Geometry check sheet. Reference: the model listing, model coordinates, mm. Give positions to 0.01 mm unless a question says otherwise; leave off trailing zeros. Loops run counter-clockwise (first coordinate to the right, second up) from the corner with the lowest first, then second, coordinate; pieces in that order, holes last. Notation, with made-up numbers: (81, 36) - (86, 36) arc R29 ccw to (86, 62) - close; hole circle Ø2 at (89, 58). An arc over 180 degrees is marked (long way). Use a Markdown table: item, result. Add a question column.
1. Cross-section at B-B on y = 2.55. Enter the section's corners in (x, z).
2. Draft check along Y on faces 1 (the flat face through (11.999, 1, 12)), 2 (the cylindrical face through (6.7, 8.06, 12.32)). Enter one of: pulls with the +Y half, pulls with the -Y half, needs draft (parallel to the pull), parting line crosses it, or undercut.
3. Cross-section at A-A on x = 2.25. Enter the section's corners in (y, z), and give its area (3 significant figures).
4. Depth check by flat-ended pin: P1, Ø12, axis at x = 2.5, y = 9, coming from the -Z side; P2, Ø0.9, axis at x = 4.75, y = 5.05, coming from the -Z side. Enter the tip coordinate at first touch or a pass-through.
5. Cross-section at C-C on z = 14.5. Count the separate pieces of the cut face and the enclosed holes in it, and give its area (3 significant figures).
from build123d import *

# Parameters (mm, degrees)
F0_W     = 22
F0_H     = 22
F0_R     = 0.75
F1_DEPTH = 25


with BuildPart() as f1:
    # F0 (on Top) → F1 (new body)
    with BuildSketch(Plane.XY):
        with Locations((0.99929, 1.25)):
            Rectangle(F0_W, F0_H)
        with Locations((-5.25, -4.95)):
            Circle(F0_R, mode=Mode.SUBTRACT)
        with Locations((-2.75, -4.95)):
            Circle(F0_R, mode=Mode.SUBTRACT)
        with Locations((-0.25, -4.95)):
            Circle(F0_R, mode=Mode.SUBTRACT)
        with Locations((-5.25, -2.45)):
            Circle(F0_R, mode=Mode.SUBTRACT)
        with Locations((-5.25, 0.05)):
            Circle(F0_R, mode=Mode.SUBTRACT)
        with Locations((-2.75, -2.45)):
            Circle(F0_R, mode=Mode.SUBTRACT)
        with Locations((-0.25, -2.45)):
            Circle(F0_R, mode=Mode.SUBTRACT)
        with Locations((-2.75, 0.05)):
            Circle(F0_R, mode=Mode.SUBTRACT)
        with Locations((-0.25, 0.05)):
            Circle(F0_R, mode=Mode.SUBTRACT)
        with Locations((2.25, -4.95)):
            Circle(F0_R, mode=Mode.SUBTRACT)
        with Locations((4.75, -4.95)):
            Circle(F0_R, mode=Mode.SUBTRACT)
        with Locations((7.25, -4.95)):
            Circle(F0_R, mode=Mode.SUBTRACT)
        with Locations((2.25, -2.45)):
            Circle(F0_R, mode=Mode.SUBTRACT)
        with Locations((4.75, -2.45)):
            Circle(F0_R, mode=Mode.SUBTRACT)
        with Locations((2.25, 0.05)):
            Circle(F0_R, mode=Mode.SUBTRACT)
        with Locations((4.75, 0.05)):
            Circle(F0_R, mode=Mode.SUBTRACT)
        with Locations((7.25, -2.45)):
            Circle(F0_R, mode=Mode.SUBTRACT)
        with Locations((7.25, 0.05)):
            Circle(F0_R, mode=Mode.SUBTRACT)
        with Locations((-5.25, 2.55)):
            Circle(F0_R, mode=Mode.SUBTRACT)
        with Locations((-5.25, 5.05)):
            Circle(F0_R, mode=Mode.SUBTRACT)
        with Locations((-2.75, 2.55)):
            Circle(F0_R, mode=Mode.SUBTRACT)
        with Locations((-0.25, 2.55)):
            Circle(F0_R, mode=Mode.SUBTRACT)
        with Locations((-2.75, 5.05)):
            Circle(F0_R, mode=Mode.SUBTRACT)
        with Locations((-0.25, 5.05)):
            Circle(F0_R, mode=Mode.SUBTRACT)
        with Locations((-5.25, 7.55)):
            Circle(F0_R, mode=Mode.SUBTRACT)
        with Locations((-2.75, 7.55)):
            Circle(F0_R, mode=Mode.SUBTRACT)
        with Locations((-0.25, 7.55)):
            Circle(F0_R, mode=Mode.SUBTRACT)
        with Locations((2.25, 2.55)):
            Circle(F0_R, mode=Mode.SUBTRACT)
        with Locations((4.75, 2.55)):
            Circle(F0_R, mode=Mode.SUBTRACT)
        with Locations((2.25, 5.05)):
            Circle(F0_R, mode=Mode.SUBTRACT)
        with Locations((4.75, 5.05)):
            Circle(F0_R, mode=Mode.SUBTRACT)
        with Locations((7.25, 2.55)):
            Circle(F0_R, mode=Mode.SUBTRACT)
        with Locations((7.25, 5.05)):
            Circle(F0_R, mode=Mode.SUBTRACT)
        with Locations((2.25, 7.55)):
            Circle(F0_R, mode=Mode.SUBTRACT)
        with Locations((4.75, 7.55)):
            Circle(F0_R, mode=Mode.SUBTRACT)
        with Locations((7.25, 7.55)):
            Circle(F0_R, mode=Mode.SUBTRACT)
    extrude(amount=F1_DEPTH)


solid = f1.part
Values found:
| question | item | result |
|---|---|---|
| 1 | outline | (-10, 0) - (-6, 0) - (-6, 25) - (-10, 25) - close; (-4.5, 0) - (-3.5, 0) - (-3.5, 25) - (-4.5, 25) - close; (-2, 0) - (-1, 0) - (-1, 25) - (-2, 25) - close; (0.5, 0) - (1.5, 0) - (1.5, 25) - (0.5, 25) - close; (3, 0) - (4, 0) - (4, 25) - (3, 25) - close; (5.5, 0) - (6.5, 0) - (6.5, 25) - (5.5, 25) - close; (8, 0) - (12, 0) - (12, 25) - (8, 25) - close |
| 2 | face 1 | needs draft |
| 2 | face 2 | undercut |
| 3 | outline | (-9.75, 0) - (-5.7, 0) - (-5.7, 25) - (-9.75, 25) - close; (-4.2, 0) - (-3.2, 0) - (-3.2, 25) - (-4.2, 25) - close; (-1.7, 0) - (-0.7, 0) - (-0.7, 25) - (-1.7, 25) - close; (0.8, 0) - (1.8, 0) - (1.8, 25) - (0.8, 25) - close; (3.3, 0) - (4.3, 0) - (4.3, 25) - (3.3, 25) - close; (5.8, 0) - (6.8, 0) - (6.8, 25) - (5.8, 25) - close; (8.3, 0) - (12.25, 0) - (12.25, 25) - (8.3, 25) - close |
| 3 | area | 325 mm2 |
| 4 | P1 | stops at z = 0 |
| 4 | P2 | passes through |
| 5 | separate pieces | 1 |
| 5 | enclosed holes | 36 |
| 5 | area | 420 mm2 |
